from build123d import *

# Parameters (mm, degrees)
F1_DEPTH = 25


with BuildPart() as f1:
    # F0 (on Front) → F1 (new body)
    with BuildSketch(Plane.XZ):
        with BuildLine():
            Line((-46.907052, 32.831196), (-49.407052, 32.831196))
            ThreePointArc((-49.407052, 32.831196), (-52.942586, 31.36673), (-54.407052, 27.831196))
            Line((-54.407052, 27.831196), (-54.407052, -2.168804))
            ThreePointArc((-54.407052, -2.168804), (-52.942586, -5.704338), (-49.407052, -7.168804))
            Line((-49.407052, -7.168804), (35.592948, -7.168804))
            ThreePointArc((35.592948, -7.168804), (45.592948, 2.831196), (35.592948, 12.831196))
            Line((35.592948, 12.831196), (-9.407052, 12.831196))
            ThreePointArc((-9.407052, 12.831196), (-12.942586, 14.295662), (-14.407052, 17.831196))
            Line((-14.407052, 17.831196), (-14.407052, 32.831196))
            Line((-14.407052, 32.831196), (-21.907052, 32.831196))
            ThreePointArc((-21.907052, 32.831196), (-34.407052, 20.331196), (-46.907052, 32.831196))
        make_face()
    extrude(amount=F1_DEPTH)


solid = f1.part
Geometry check sheet. Reference: the model listing, model coordinates, mm. A direction names the side the tool comes from. Round coordinates to 2 decimals unless told otherwise and drop trailing zeros. Write each loop counter-clockwise with the first axis right and the second up, starting at its lowest first coordinate (ties: lowest second). Pieces come first, ordered by that corner, then holes. Notation, with made-up numbers: (-30.75, 21.5) -> (15.25, 21.5) arc R27 cw to (15.25, 47.5) -> close; hole circle Ø7 at (18, -17). An arc over 180 degrees is marked (long way). One line per item, written item: value. Start each with the question number.
(1) Go/stop test with flat-tipped pins: pin 1 Ø1.5 at (x, y) = (-28.5, -4) entering from +Z; pin 2 Ø1 at (x, y) = (-37.5, -12) entering from +Z; pin 3 Ø6 at (x, z) = (13, 11.5) entering from +Y; pin 4 Ø12 at (y, z) = (-8.5, 28.5) entering from +X. Record where each tip stops, or that it passes through.
(2) Cross-section at C-C, the plane x = -2.5. Record the cut outline in (y, z).
(3) Cross-section at D-D, the plane z = 29. Record the cut outline in (x, y), and give its area (3 significant figures).
(4) Cross-section at B-B, the plane y = -15. Record the cut outline in (x, z), and give its area (3 significant figures).
(5) Draft check along X on faces 3 (the cylindrical face through (45.59, -12.32, 2.61)), 4 (the flat face through (-18, -12, 32.831)), 5 (the cylindrical face through (-34.132, -12.325, 20.334)). Enter one of: +X half, -X half, draft (parallel to the pull), parting line (faces both ways), or undercut.
(6) Cross-section at A-A, the plane z = 21.5. Record the cut outline in (x, y).
(7) Access from +Z, -Z, +X, -X, +Y, -Y to the whole of each face (thin tool, end or side, straight path). Record for faces 1 (the flat face through (-14.407, -12, 25)), 2 (the cylindrical face through (-52.981, -12.325, -5.665)).
(8) Scan lines: line 1 (X direction, y = -6, z = 30); line 2 (Z direction, x = -4, y = -6.75); line 3 (X direction, y = -5.5, z = 28.5). Record each from-to range of solid material in increasing order. Write a range as [from, to].
Answer:
1. pin 1: z = 22.25
1. pin 2: z = 20.86
1. pin 3: y = 0
1. pin 4: x = -14.41
2. outline: (-25, -7.17) -> (0, -7.17) -> (0, 12.83) -> (-25, 12.83) -> close
3. outline: (-54.27, -25) -> (-46.31, -25) -> (-46.31, 0) -> (-54.27, 0) -> close; (-22.51, -25) -> (-14.41, -25) -> (-14.41, 0) -> (-22.51, 0) -> close
3. area: 402 mm²
4. outline: (-54.41, -2.17) arc R5 ccw to (-49.41, -7.17) -> (35.59, -7.17) arc R10 ccw to (35.59, 12.83) -> (-9.41, 12.83) arc R5 cw to (-14.41, 17.83) -> (-14.41, 32.83) -> (-21.91, 32.83) arc R12.5 cw to (-46.91, 32.83) -> (-49.41, 32.83) arc R5 ccw to (-54.41, 27.83) -> close
4. area: 2,510 mm²
5. face 3: +X half
5. face 4: draft
5. face 5: undercut
6. outline: (-54.41, -25) -> (-39.68, -25) -> (-39.68, 0) -> (-54.41, 0) -> close; (-29.13, -25) -> (-14.41, -25) -> (-14.41, 0) -> (-29.13, 0) -> close
7. face 1: +Z, +X, +Y, -Y
7. face 2: -Z, -X, +Y, -Y
8. line 1: [-53.91, -46.58], [-22.23, -14.41]
8. line 2: [-7.17, 12.83]
8. line 3: [-54.36, -46.13], [-22.68, -14.41]
